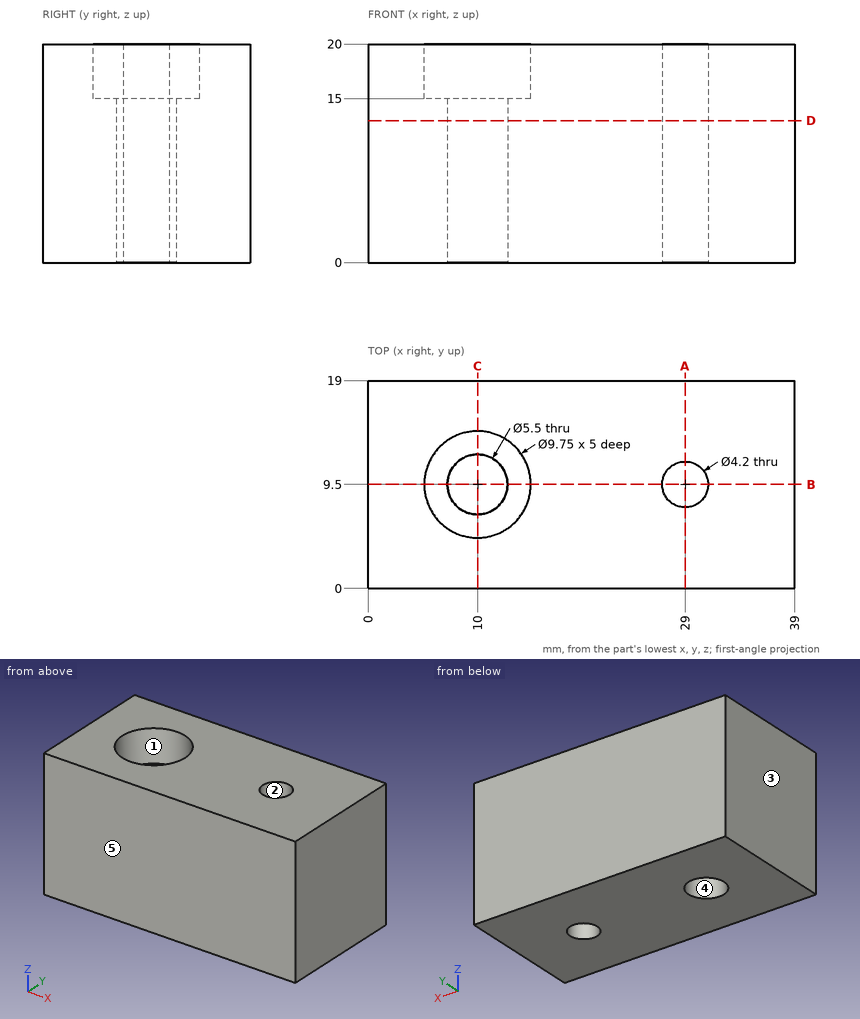
Answer from the drawing. Dimensions are ordinates in mm from the lowest x, y and z of the part. A direction names the side the tool comes from. Round coordinates to 2 decimals unless told otherwise and drop trailing zeros. Loops run counter-clockwise (first coordinate to the right, second up) from the corner with the lowest first, then second, coordinate; pieces in that order, holes last. Notation, with made-up numbers: (-8.75, -11.5) - (22.25, -11.5) arc R13 ccw to (22.25, 9.5) - close; hole circle Ø7 at (-32.5, -35.75). An arc over 180 degrees is marked (long way). One line per item, written item: value.
Q1. Find section B-B on y = 9.5. Give the vertices of the cut face in (x, z) (3 decimals).
Check values:
outline: (0, 0) - (7.25, 0) - (7.25, 15) - (5.125, 15) - (5.125, 20) - (0, 20) - close; (12.75, 0) - (26.9, 0) - (26.9, 20) - (14.875, 20) - (14.875, 15) - (12.75, 15) - close; (31.1, 0) - (39, 0) - (39, 20) - (31.1, 20) - close
Q2. Straight lines are drawn through the part: probe 1 along Y at (x, z) = (10, 11.75); probe 2 along Y at (x, z) = (10, 18.7) (3 decimals); probe 3 along X at (y, z) = (8.75, 15.5). For each, find the intervals that lie inside material, in ascending order.
Check values:
probe 1: 0 to 6.75, 12.25 to 19
probe 2: 0 to 4.625, 14.375 to 19
probe 3: 0 to 5.18, 14.82 to 27.04, 30.96 to 39
Q3. For the marked faces 1 and 2, determine the directions among +Z, -Z, +X, -X, +Y, -Y from which every point of the face is accessible in a straight line to the end or side of a thin tool.
Check values:
face 1: +Z
face 2: +Z, -Z
Q4. The mould has two halves that part along X. Classify the marked faces 3, 4 and 5: +X half, -X half, draft (parallel to the pull), parting line (faces both ways), or undercut.
Check values:
face 3: -X half
face 4: undercut
face 5: draft
Q5. Find section D-D on z = 13. Give the vertices of the cut face in (x, y), and give its area (3 significant figures).
Check values:
outline: (0, 0) - (39, 0) - (39, 19) - (0, 19) - close; hole circle Ø5.5 at (10, 9.5); hole circle Ø4.2 at (29, 9.5)
area: 703 mm2
Q6. Each of these flat-tipped pins is pushed along its axis until it touches: pin 1 Ø4 at (x, y) = (29, 9.5) entering from +Z; pin 2 Ø5 at (x, y) = (10, 11) entering from +Z. Where does it stop, or does it pass through?
Check values:
pin 1: through
pin 2: z = 15
Q7. Find section A-A on x = 29. Give the vertices of the cut face in (y, z).
Check values:
outline: (0, 0) - (7.4, 0) - (7.4, 20) - (0, 20) - close; (11.6, 0) - (19, 0) - (19, 20) - (11.6, 20) - close
Q8. Find section C-C on x = 10. Give the vertices of the cut face in (y, z) (3 decimals).
Check values:
outline: (0, 0) - (6.75, 0) - (6.75, 15) - (4.625, 15) - (4.625, 20) - (0, 20) - close; (12.25, 0) - (19, 0) - (19, 20) - (14.375, 20) - (14.375, 15) - (12.25, 15) - close
